```python
from build123d import *

# Parameters (mm, degrees)
SKETCH2_W                                        = 110
SKETCH2_H                                        = 55
BOSS_EXTRUDE1_DEPTH                              = 80
SKETCH4_W                                        = 90
SKETCH4_H                                        = 60
CUT_EXTRUDE2_DEPTH                               = 10
CUT_EXTRUDE2_DRAFT                               = -20
CBORE_FOR_M6_HEX_HEAD_MACHINE_SCREW1_D           = 7
CBORE_FOR_M6_HEX_HEAD_MACHINE_SCREW1_CBORE_D     = 13.95
CBORE_FOR_M6_HEX_HEAD_MACHINE_SCREW1_CBORE_DEPTH = 4.7
SHELL4_START                                     = 15
SHELL4_OUTLINE_W                                 = 100
SHELL4_OUTLINE_H                                 = 75
SHELL4_OUTLINE_R                                 = 11.975
SHELL4_DEPTH                                     = 35
SHELL4_2_OUTLINE_R                               = 11.975
SHELL4_2_OUTLINE_R_2                             = 8.5
SHELL4_2_DEPTH                                   = 30.3
SHELL4_3_OUTLINE_W                               = 100
SHELL4_3_OUTLINE_H                               = 10
SHELL4_3_DEPTH                                   = 2.859259966
SHELL4_4_DEPTH                                   = 75
SHELL4_START_2                                   = 5
SHELL4_5_DEPTH                                   = 100
CUT_EXTRUDE4_REACH                               = 146.049
SKETCH8_R                                        = 2.5
SKETCH8_R_2                                      = 4


with BuildPart() as part:
    # Sketch2 → Boss-Extrude1 (new body)
    with BuildSketch(Plane.XY):
        with Locations((55, 27.5)):
            Rectangle(SKETCH2_W, SKETCH2_H)
    extrude(amount=BOSS_EXTRUDE1_DEPTH)


with BuildPart() as cut_extrude2_tool:
    # Sketch4 → Cut-Extrude2 (with draft: the straight prism first)
    with BuildSketch(Plane(origin=(0, 10, 0), x_dir=(-1, 0, 0), z_dir=(0, -1, 0))):
        with Locations((-55, -40)):
            Rectangle(SKETCH4_W, SKETCH4_H)
    extrude(amount=CUT_EXTRUDE2_DEPTH)
    # Cut-Extrude2: the draft: its side faces are tilted about the plane it starts from
    cut_extrude2_sides = [cut_extrude2_tool.faces().sort_by_distance(p)[0] for p in [
        (55, 5, 70),
        (10, 5, 40),
        (55, 5, 10),
        (100, 5, 40),
    ]]
    draft(cut_extrude2_sides, Plane(origin=(0, 10, 0), x_dir=(-1, 0, 0), z_dir=(0, -1, 0)), CUT_EXTRUDE2_DRAFT)


with BuildPart() as part_1:
    add(part.part)

    # Cut-Extrude2: cut by cut_extrude2_tool
    add(cut_extrude2_tool.part, mode=Mode.SUBTRACT)

    # CBORE for M6 Hex Head Machine Screw1 (through all)
    with Locations(Plane(origin=(0, 55, 0), x_dir=(1, 0, 0), z_dir=(0, 1, 0))):
        with Locations((55, -40)):
            CounterBoreHole(CBORE_FOR_M6_HEX_HEAD_MACHINE_SCREW1_D / 2, CBORE_FOR_M6_HEX_HEAD_MACHINE_SCREW1_CBORE_D / 2, CBORE_FOR_M6_HEX_HEAD_MACHINE_SCREW1_CBORE_DEPTH)

    # Shell4: read off the stored shape, not the designer's step
    # Shell4 outline → Shell4 (cut)
    with BuildSketch(Plane(origin=(0, 0, 0), x_dir=(1, 0, 0), z_dir=(0, 1, 0)).offset(SHELL4_START)):
        with Locations((55, -37.5)):
            Rectangle(SHELL4_OUTLINE_W, SHELL4_OUTLINE_H)
        with Locations((55, -40)):
            Circle(SHELL4_OUTLINE_R, mode=Mode.SUBTRACT)
    extrude(amount=SHELL4_DEPTH, mode=Mode.SUBTRACT)

    # Shell4 2 outline → Shell4 2 (cut)
    with BuildSketch(Plane(origin=(0, 0, 0), x_dir=(1, 0, 0), z_dir=(0, 1, 0)).offset(SHELL4_START)):
        with Locations((55, -40)):
            Circle(SHELL4_2_OUTLINE_R)
        with Locations((55, -40)):
            Circle(SHELL4_2_OUTLINE_R_2, mode=Mode.SUBTRACT)
    extrude(amount=SHELL4_2_DEPTH, mode=Mode.SUBTRACT)

    # Shell4 3 outline → Shell4 3 (cut)
    with BuildSketch(Plane.XY):
        with Locations((55, 10)):
            Rectangle(SHELL4_3_OUTLINE_W, SHELL4_3_OUTLINE_H)
    extrude(amount=SHELL4_3_DEPTH, mode=Mode.SUBTRACT)

    # Shell4 4 outline → Shell4 4 (cut)
    with BuildSketch(Plane.XY):
        Polygon((103.501037691, 15), (105, 10.881634904), (105, 15), align=None)
        Polygon((5, 15), (5, 10.881634904), (6.498962309, 15), align=None)
    extrude(amount=SHELL4_4_DEPTH, mode=Mode.SUBTRACT)

    # Shell4 5 outline → Shell4 5 (cut)
    with BuildSketch(Plane.YZ.offset(SHELL4_START_2)):
        Polygon((15, 2.859259966), (15, 6.498962309), (5, 2.859259966), align=None)
        Polygon((15, 75), (10.881634904, 75), (15, 73.501037691), align=None)
    extrude(amount=SHELL4_5_DEPTH, mode=Mode.SUBTRACT)

    # Sketch8 → Cut-Extrude4 (cut, up to next)
    with BuildSketch(Plane(origin=(0, 0, 75), x_dir=(-1, 0, 0), z_dir=(0, 0, -1)), mode=Mode.PRIVATE) as cut_extrude4_sk1:
        with Locations((-97, 31)):
            Circle(SKETCH8_R)
    cut_extrude4_tool1 = extrude(cut_extrude4_sk1.sketch, amount=-CUT_EXTRUDE4_REACH, mode=Mode.PRIVATE) & part_1.part
    # Sketch8 → Cut-Extrude4 (cut, up to next)
    with BuildSketch(Plane(origin=(0, 0, 75), x_dir=(-1, 0, 0), z_dir=(0, 0, -1)), mode=Mode.PRIVATE) as cut_extrude4_sk2:
        with Locations((-97, 23)):
            Circle(SKETCH8_R_2)
    cut_extrude4_tool2 = extrude(cut_extrude4_sk2.sketch, amount=-CUT_EXTRUDE4_REACH, mode=Mode.PRIVATE) & part_1.part
    # Sketch8 → Cut-Extrude4 (cut, up to next)
    with BuildSketch(Plane(origin=(0, 0, 75), x_dir=(-1, 0, 0), z_dir=(0, 0, -1)), mode=Mode.PRIVATE) as cut_extrude4_sk3:
        with Locations((-86.5, 31)):
            Circle(SKETCH8_R)
    cut_extrude4_tool3 = extrude(cut_extrude4_sk3.sketch, amount=-CUT_EXTRUDE4_REACH, mode=Mode.PRIVATE) & part_1.part
    # Sketch8 → Cut-Extrude4 (cut, up to next)
    with BuildSketch(Plane(origin=(0, 0, 75), x_dir=(-1, 0, 0), z_dir=(0, 0, -1)), mode=Mode.PRIVATE) as cut_extrude4_sk4:
        with Locations((-86.5, 23)):
            Circle(SKETCH8_R_2)
    cut_extrude4_tool4 = extrude(cut_extrude4_sk4.sketch, amount=-CUT_EXTRUDE4_REACH, mode=Mode.PRIVATE) & part_1.part
    # Sketch8 → Cut-Extrude4 (cut, up to next)
    with BuildSketch(Plane(origin=(0, 0, 75), x_dir=(-1, 0, 0), z_dir=(0, 0, -1)), mode=Mode.PRIVATE) as cut_extrude4_sk5:
        with Locations((-76, 31)):
            Circle(SKETCH8_R)
    cut_extrude4_tool5 = extrude(cut_extrude4_sk5.sketch, amount=-CUT_EXTRUDE4_REACH, mode=Mode.PRIVATE) & part_1.part
    # Sketch8 → Cut-Extrude4 (cut, up to next)
    with BuildSketch(Plane(origin=(0, 0, 75), x_dir=(-1, 0, 0), z_dir=(0, 0, -1)), mode=Mode.PRIVATE) as cut_extrude4_sk6:
        with Locations((-76, 23)):
            Circle(SKETCH8_R_2)
    cut_extrude4_tool6 = extrude(cut_extrude4_sk6.sketch, amount=-CUT_EXTRUDE4_REACH, mode=Mode.PRIVATE) & part_1.part
    # Sketch8 → Cut-Extrude4 (cut, up to next)
    with BuildSketch(Plane(origin=(0, 0, 75), x_dir=(-1, 0, 0), z_dir=(0, 0, -1)), mode=Mode.PRIVATE) as cut_extrude4_sk7:
        with Locations((-65.5, 31)):
            Circle(SKETCH8_R)
    cut_extrude4_tool7 = extrude(cut_extrude4_sk7.sketch, amount=-CUT_EXTRUDE4_REACH, mode=Mode.PRIVATE) & part_1.part
    # Sketch8 → Cut-Extrude4 (cut, up to next)
    with BuildSketch(Plane(origin=(0, 0, 75), x_dir=(-1, 0, 0), z_dir=(0, 0, -1)), mode=Mode.PRIVATE) as cut_extrude4_sk8:
        with Locations((-65.5, 23)):
            Circle(SKETCH8_R_2)
    cut_extrude4_tool8 = extrude(cut_extrude4_sk8.sketch, amount=-CUT_EXTRUDE4_REACH, mode=Mode.PRIVATE) & part_1.part
    # Sketch8 → Cut-Extrude4 (cut, up to next)
    with BuildSketch(Plane(origin=(0, 0, 75), x_dir=(-1, 0, 0), z_dir=(0, 0, -1)), mode=Mode.PRIVATE) as cut_extrude4_sk9:
        with Locations((-55, 31)):
            Circle(SKETCH8_R)
    cut_extrude4_tool9 = extrude(cut_extrude4_sk9.sketch, amount=-CUT_EXTRUDE4_REACH, mode=Mode.PRIVATE) & part_1.part
    # Sketch8 → Cut-Extrude4 (cut, up to next)
    with BuildSketch(Plane(origin=(0, 0, 75), x_dir=(-1, 0, 0), z_dir=(0, 0, -1)), mode=Mode.PRIVATE) as cut_extrude4_sk10:
        with Locations((-55, 23)):
            Circle(SKETCH8_R_2)
    cut_extrude4_tool10 = extrude(cut_extrude4_sk10.sketch, amount=-CUT_EXTRUDE4_REACH, mode=Mode.PRIVATE) & part_1.part
    # Sketch8 → Cut-Extrude4 (cut, up to next)
    with BuildSketch(Plane(origin=(0, 0, 75), x_dir=(-1, 0, 0), z_dir=(0, 0, -1)), mode=Mode.PRIVATE) as cut_extrude4_sk11:
        with Locations((-44.5, 31)):
            Circle(SKETCH8_R)
    cut_extrude4_tool11 = extrude(cut_extrude4_sk11.sketch, amount=-CUT_EXTRUDE4_REACH, mode=Mode.PRIVATE) & part_1.part
    # Sketch8 → Cut-Extrude4 (cut, up to next)
    with BuildSketch(Plane(origin=(0, 0, 75), x_dir=(-1, 0, 0), z_dir=(0, 0, -1)), mode=Mode.PRIVATE) as cut_extrude4_sk12:
        with Locations((-44.5, 23)):
            Circle(SKETCH8_R_2)
    cut_extrude4_tool12 = extrude(cut_extrude4_sk12.sketch, amount=-CUT_EXTRUDE4_REACH, mode=Mode.PRIVATE) & part_1.part
    # Sketch8 → Cut-Extrude4 (cut, up to next)
    with BuildSketch(Plane(origin=(0, 0, 75), x_dir=(-1, 0, 0), z_dir=(0, 0, -1)), mode=Mode.PRIVATE) as cut_extrude4_sk13:
        with Locations((-34, 31)):
            Circle(SKETCH8_R)
    cut_extrude4_tool13 = extrude(cut_extrude4_sk13.sketch, amount=-CUT_EXTRUDE4_REACH, mode=Mode.PRIVATE) & part_1.part
    # Sketch8 → Cut-Extrude4 (cut, up to next)
    with BuildSketch(Plane(origin=(0, 0, 75), x_dir=(-1, 0, 0), z_dir=(0, 0, -1)), mode=Mode.PRIVATE) as cut_extrude4_sk14:
        with Locations((-34, 23)):
            Circle(SKETCH8_R_2)
    cut_extrude4_tool14 = extrude(cut_extrude4_sk14.sketch, amount=-CUT_EXTRUDE4_REACH, mode=Mode.PRIVATE) & part_1.part
    # Sketch8 → Cut-Extrude4 (cut, up to next)
    with BuildSketch(Plane(origin=(0, 0, 75), x_dir=(-1, 0, 0), z_dir=(0, 0, -1)), mode=Mode.PRIVATE) as cut_extrude4_sk15:
        with Locations((-23.5, 31)):
            Circle(SKETCH8_R)
    cut_extrude4_tool15 = extrude(cut_extrude4_sk15.sketch, amount=-CUT_EXTRUDE4_REACH, mode=Mode.PRIVATE) & part_1.part
    # Sketch8 → Cut-Extrude4 (cut, up to next)
    with BuildSketch(Plane(origin=(0, 0, 75), x_dir=(-1, 0, 0), z_dir=(0, 0, -1)), mode=Mode.PRIVATE) as cut_extrude4_sk16:
        with Locations((-23.5, 23)):
            Circle(SKETCH8_R_2)
    cut_extrude4_tool16 = extrude(cut_extrude4_sk16.sketch, amount=-CUT_EXTRUDE4_REACH, mode=Mode.PRIVATE) & part_1.part
    # Sketch8 → Cut-Extrude4 (cut, up to next)
    with BuildSketch(Plane(origin=(0, 0, 75), x_dir=(-1, 0, 0), z_dir=(0, 0, -1)), mode=Mode.PRIVATE) as cut_extrude4_sk17:
        with Locations((-13, 31)):
            Circle(SKETCH8_R)
    cut_extrude4_tool17 = extrude(cut_extrude4_sk17.sketch, amount=-CUT_EXTRUDE4_REACH, mode=Mode.PRIVATE) & part_1.part
    # Sketch8 → Cut-Extrude4 (cut, up to next)
    with BuildSketch(Plane(origin=(0, 0, 75), x_dir=(-1, 0, 0), z_dir=(0, 0, -1)), mode=Mode.PRIVATE) as cut_extrude4_sk18:
        with Locations((-13, 23)):
            Circle(SKETCH8_R_2)
    cut_extrude4_tool18 = extrude(cut_extrude4_sk18.sketch, amount=-CUT_EXTRUDE4_REACH, mode=Mode.PRIVATE) & part_1.part
    add(cut_extrude4_tool1.solids().sort_by_distance((97, 31, 75))[0], mode=Mode.SUBTRACT)
    add(cut_extrude4_tool2.solids().sort_by_distance((97, 23, 75))[0], mode=Mode.SUBTRACT)
    add(cut_extrude4_tool3.solids().sort_by_distance((86.5, 31, 75))[0], mode=Mode.SUBTRACT)
    add(cut_extrude4_tool4.solids().sort_by_distance((86.5, 23, 75))[0], mode=Mode.SUBTRACT)
    add(cut_extrude4_tool5.solids().sort_by_distance((76, 31, 75))[0], mode=Mode.SUBTRACT)
    add(cut_extrude4_tool6.solids().sort_by_distance((76, 23, 75))[0], mode=Mode.SUBTRACT)
    add(cut_extrude4_tool7.solids().sort_by_distance((65.5, 31, 75))[0], mode=Mode.SUBTRACT)
    add(cut_extrude4_tool8.solids().sort_by_distance((65.5, 23, 75))[0], mode=Mode.SUBTRACT)
    add(cut_extrude4_tool9.solids().sort_by_distance((55, 31, 75))[0], mode=Mode.SUBTRACT)
    add(cut_extrude4_tool10.solids().sort_by_distance((55, 23, 75))[0], mode=Mode.SUBTRACT)
    add(cut_extrude4_tool11.solids().sort_by_distance((44.5, 31, 75))[0], mode=Mode.SUBTRACT)
    add(cut_extrude4_tool12.solids().sort_by_distance((44.5, 23, 75))[0], mode=Mode.SUBTRACT)
    add(cut_extrude4_tool13.solids().sort_by_distance((34, 31, 75))[0], mode=Mode.SUBTRACT)
    add(cut_extrude4_tool14.solids().sort_by_distance((34, 23, 75))[0], mode=Mode.SUBTRACT)
    add(cut_extrude4_tool15.solids().sort_by_distance((23.5, 31, 75))[0], mode=Mode.SUBTRACT)
    add(cut_extrude4_tool16.solids().sort_by_distance((23.5, 23, 75))[0], mode=Mode.SUBTRACT)
    add(cut_extrude4_tool17.solids().sort_by_distance((13, 31, 75))[0], mode=Mode.SUBTRACT)
    add(cut_extrude4_tool18.solids().sort_by_distance((13, 23, 75))[0], mode=Mode.SUBTRACT)


solid = part_1.part
```
The model under review builds one solid part; all positions refer to its coordinate system, in mm. A direction names the side the tool comes from. Coordinates: 2 decimals unless noted, no trailing zeros. Write each loop counter-clockwise with the first axis right and the second up, starting at its lowest first coordinate (ties: lowest second). Pieces come first, ordered by that corner, then holes. Notation, with made-up numbers: (34.25, 28.25) - (84.25, 28.25) arc R17 ccw to (84.25, 47.25) - close; hole circle Ø4 at (-10.75, -18.75). An arc over 180 degrees is marked (long way). Write item = value, one per line.
(1) Consider section B-B, the plane z = 56. Give the boundary of the cut face in (x, y), then the cut area to 3 significant figures.
Result sheet:
outline = (0, 0) - (6.36, 0) - (10, 10) - (100, 10) - (103.64, 0) - (110, 0) - (110, 55) - (0, 55) - close; hole (5, 10.88) - (6.5, 15) - (103.5, 15) - (105, 10.88) - (105, 50) - (5, 50) - close
area = 1,610 mm^2
(2) For P1, Ø6.5, axis at x = 76, y = 23, coming from the +Z side; P2, Ø1.5, axis at x = 12.5, y = 14.5, coming from the -Z side; P3, Ø4, axis at x = 54.5, z = 41.5, coming from the +Y side; P4, Ø3, axis at x = 87, y = 14, coming from the -Z side, all flat-tipped, find the tip position at first contact; note any pin that passes through.
Result sheet:
P1 = through
P2 = 6.04
P3 = 50.3
P4 = 5.59
(3) Consider section A-A, the plane y = 48.5. Give the boundary of the cut face in (x, z) (3 decimals), then the cut area to 3 significant figures.
Result sheet:
outline = (0, 0) - (5, 0) - (5, 75) - (105, 75) - (105, 0) - (110, 0) - (110, 80) - (0, 80) - close; circle Ø23.95 at (55, 40); hole circle Ø7 at (55, 40)
area = 1,710 mm^2
(4) Consider section D-D, the plane z = 40. State how many separate pieces and enclosed holes the cut face has, then the cut area to 3 significant figures.
Result sheet:
separate_pieces = 2
enclosed_holes = 2
area = 1,890 mm^2
(5) Machinability: for faces 1 (the face through (54, 55, 48)), 2 (the face through (54.3, 12.91, 74.26)), 3 (the face through (45.021, 26.966, 77.465)), 4 (the face through (14.84, 32.69, 77.46)), 5 (the face through (56, 10, 33)), which of the approach directions +Z, -Z, +X, -X, +Y, -Y give a long, thin tool a straight path to every point of the face, cutting with its end or side? Answer none if there is none.
Result sheet:
face_1 = +Z, -Z, +X, -X, +Y
face_2 = none
face_3 = +Z
face_4 = +Z, -Z
face_5 = -Y
(6) Mouldability with a two-part tool opening along X and no side actions: class faces 6 (the face through (97.521, 26.966, 77.465)), 7 (the face through (43, 0, 75)), 8 (the face through (87.021, 26.966, 77.465)), 9 (the face through (110, 27, 39)) as pulls with the +X half, pulls with the -X half, needs draft (parallel to the pull), parting line crosses it, or undercut.
Result sheet:
face_6 = undercut
face_7 = needs draft
face_8 = undercut
face_9 = pulls with the +X half
(7) For line 1 (Y direction, x = 34, z = 76.9); line 2 (Y direction, x = 76.5, z = 63); line 3 (X direction, y = 34, z = 14), list the stretches that pass through material, from the lowest coordinate up. Write a range as [from, to].
Result sheet:
line_1 = [0, 19], [27, 28.5], [33.5, 55]
line_2 = [10, 15], [50, 55]
line_3 = [0, 5], [105, 110]
(8) Consider section C-C, the plane x = 86.5. Give the boundary of the cut face in (y, z), then the cut area to 3 significant figures.
Result sheet:
outline = (0, 0) - (5, 0) - (5, 2.86) - (15, 6.5) - (15, 73.5) - (10.88, 75) - (19, 75) - (19, 80) - (0, 80) - (0, 73.64) - (10, 70) - (10, 10) - (0, 6.36) - close; (27, 75) - (28.5, 75) - (28.5, 80) - (27, 80) - close; (33.5, 75) - (50, 75) - (50, 0) - (55, 0) - (55, 80) - (33.5, 80) - close
area = 1,020 mm^2
